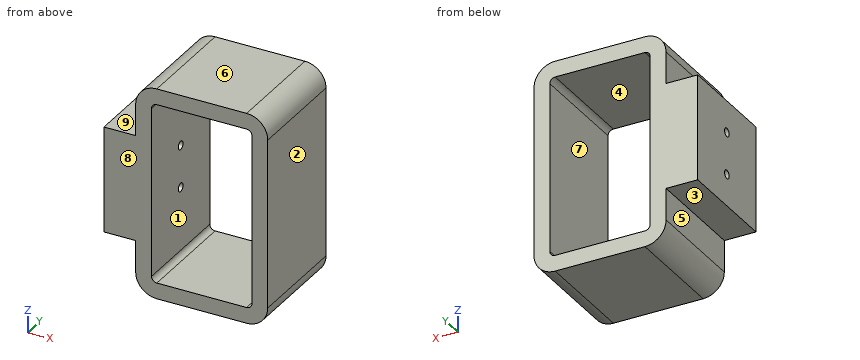
Autodesk Fusion 360 part; units mm, degrees
sketch "Sketch1" plane through (0, 0, 0) normal (1, 0, 0) x (0, 0, -1)
sketch "Sketch2" plane through (0, 0, 0) normal (0, 1, 0) x (1, 0, 0)
  line L0 (10, 0) -> (52.5, 0)
  line L1 (62.5, -10) -> (62.5, -90)
  line L2 (52.5, -100) -> (10, -100)
  line L3 (0, -25) -> (-15, -25)
  line L4 (-15, -25) -> (-15, -75)
  line L5 (-15, -75) -> (0, -75)
  arc A0 (10, 0) -> (0, -10) centre (10, -10) ccw
  arc A1 (62.5, -10) -> (52.5, 0) centre (52.5, -10) ccw
  arc A2 (52.5, -100) -> (62.5, -90) centre (52.5, -90) ccw
  arc A3 (0, -90) -> (10, -100) centre (10, -90) ccw
  arc A4 (10, -7.5) -> (7.5, -10) centre (10, -10) ccw
  line L6 (7.5, -90) -> (7.5, -10)
  arc A5 (7.5, -90) -> (10, -92.5) centre (10, -90) ccw
  line L7 (52.5, -92.5) -> (10, -92.5)
  arc A6 (52.5, -92.5) -> (55, -90) centre (52.5, -90) ccw
  line L8 (55, -10) -> (55, -90)
  arc A7 (55, -10) -> (52.5, -7.5) centre (52.5, -10) ccw
  line L9 (10, -7.5) -> (52.5, -7.5)
  line L10 (0, -90) -> (0, -75)
  line L11 (0, -25) -> (0, -10)
  point P0 (62.5, 0)
  point P1 (0, -100)
extrude "Extrude1" add sketch "Sketch2" along normal blind 50
sketch "Sketch3" plane through (-15, 0, 0) normal (-1, 0, 0) x (0, 0, 1)
  line L0 (25, 0) -> (75, 0)
  line L1 (75, 0) -> (75, 50)
  line L2 (75, 50) -> (25, 50)
  line L3 (25, 50) -> (25, 0)
  circle A0 centre (40, 25) radius 2
  circle A1 centre (60, 25) radius 2
  dimension "d7" = 4
  dimension "d8" = 4
extrude "Extrude2" cut sketch "Sketch3" against normal blind 45 contours A0 | A1
Design review of the part built by this model. Coordinates are the model's own, in mm. Face numbers are marked on the shaded views. A direction names the side the tool comes from. Give positions to 0.01 mm unless a question says otherwise; leave off trailing zeros. Loops run counter-clockwise (first coordinate to the right, second up) from the corner with the lowest first, then second, coordinate; pieces in that order, holes last. Notation, with made-up numbers: M 43.5,27 L 63.5,27 A15 ccw 63.5,32 Z; hole C -28.5,11 d9. An arc over 180 degrees is marked long. One line per question, with ' | ' between items. Start each with the question number.
1. Add section A-A (z = 20). Write out the cut boundary in (x, y), plus the area to 3 significant figures.
2. Add section C-C (z = 60). Write out the cut boundary in (x, y).
3. Insertion check: P1, Ø16.5, axis at y = 19, z = 16, coming from the -X side; P2, Ø12, axis at x = -6.5, y = 22, coming from the +Z side; P3, Ø16.5, axis at x = -9.5, y = 30.5, coming from the -Z side. Each pin has a flat end and moves straight along its axis. Give the tip position at first contact, or say it passes through.
4. Add section D-D (x = -3.5). Write out the cut boundary in (y, z).
5. Add section B-B (y = 25). Write out the cut boundary in (x, z), plus the area to 3 significant figures.
6. For the marked faces 5, 6, 7, 8 and 9, list the 3-axis set-ups (+Z, -Z, +X, -X, +Y, -Y) from which the entire face can be reached by the end or side of a thin tool; tool diameter is ignored.
7. To check wall thickness, follow L1, parallel to X at y = 32.5, z = 78.5; L2, parallel to Z at x = 42.5, y = 14; L3, parallel to X at y = 19, z = 42. State the ranges of each line that lie inside material, in increasing order.
8. The part is to be moulded in two halves that separate along Z. For the marked faces 1, 2, 3 and 4, say which applies: released by +Z, released by -Z, zero draft, split by the parting line, or undercut.
Worked out:
1) outline: M 0,0 L 7.5,0 L 7.5,50 L 0,50 Z; M 55,0 L 62.5,0 L 62.5,50 L 55,50 Z | area: 750 mm²
2) outline: M -15,0 L 7.5,0 L 7.5,23 L -15,23 Z; M -15,27 L 7.5,27 L 7.5,50 L -15,50 Z; M 55,0 L 62.5,0 L 62.5,50 L 55,50 Z
3) P1: stops at x = 0 | P2: stops at z = 75 | P3: stops at z = 25
4) outline: M 0,25 L 50,25 L 50,75 L 0,75 Z; hole C 25,40 d4; hole C 25,60 d4
5) outline: M -15,25 L 0,25 L 0,10 A10 ccw 10,0 L 52.5,0 A10 ccw 62.5,10 L 62.5,90 A10 ccw 52.5,100 L 10,100 A10 ccw 0,90 L 0,75 L -15,75 L -15,62 L 7.5,62 L 7.5,90 A2.5 cw 10,92.5 L 52.5,92.5 A2.5 cw 55,90 L 55,10 A2.5 cw 52.5,7.5 L 10,7.5 A2.5 cw 7.5,10 L 7.5,38 L -15,38 Z; M -15,42 L 7.5,42 L 7.5,58 L -15,58 Z | area: 2,700 mm²
6) face 5: -Z, -X, +Y, -Y | face 6: +Z, +X, -X, +Y, -Y | face 7: +Y, -Y | face 8: +Z, -Z, +X, -X, -Y | face 9: +Z, -X, +Y, -Y
7) L1: x = 0 to 7.5, 55 to 62.5 | L2: z = 0 to 7.5, 92.5 to 100 | L3: x = -15 to 7.5, 55 to 62.5
8) face 1: undercut | face 2: zero draft | face 3: released by -Z | face 4: undercut
